from build123d import *

# Parameters (mm, degrees)
F0_W     = 380
F0_H     = 380
F1_DEPTH = 380
F2_W     = 342
F2_H     = 342
F3_DEPTH = 361
F4_W     = 40
F4_H     = 40
F5_DEPTH = 150


with BuildPart() as f1:
    # F0 (on Top) → F1 (new body)
    with BuildSketch(Plane.XY):
        Rectangle(F0_W, F0_H)
    extrude(amount=F1_DEPTH)

    # F2 (on face) → F3 (cut)
    with BuildSketch(Plane(origin=(-190, 0, 0), x_dir=(0, -1, 0), z_dir=(-1, 0, 0))):
        with Locations((0, 190)):
            Rectangle(F2_W, F2_H)
    extrude(amount=-F3_DEPTH, mode=Mode.SUBTRACT)

    # F4 (on face) → F5 (join)
    with BuildSketch(Plane(origin=(0, 0, 0), x_dir=(1, 0, 0), z_dir=(0, 0, -1))):
        with Locations((170, 170)):
            Rectangle(F4_W, F4_H)
        with Locations((-170, 170)):
            Rectangle(F4_W, F4_H)
        with Locations((-170, -170)):
            Rectangle(F4_W, F4_H)
        with Locations((170, -170)):
            Rectangle(F4_W, F4_H)
    extrude(amount=F5_DEPTH)


solid = f1.part
Source: CAD feature listing. Evaluate the final solid. Frame: model axes, mm. A direction names the side the tool comes from. Give positions to 0.01 mm unless a question says otherwise; leave off trailing zeros. Write each loop counter-clockwise with the first axis right and the second up, starting at its lowest first coordinate (ties: lowest second). Pieces come first, ordered by that corner, then holes. Notation, with made-up numbers: M 34,1 L 91,1 A26 ccw 91,26 Z; hole C 16,57.5 d10. An arc over 180 degrees is marked long. Answer as a JSON object with one key per item and string values.
Q1. Contact query for flat-ended pins moving along their axis: P1, Ø1, axis at y = -9.5, z = 195.5, coming from the -X side; P2, Ø3, axis at x = 116, y = -54.5, coming from the -Z side. Output: stop coordinate, or through.
Geometry check:
{"P1": "stops at x = 171", "P2": "stops at z = 0"}
Q2. Ray query, line 1 along Y through (x, z) = (152.5, 319); line 2 along X through (y, z) = (-154, -49.5); line 3 along Z through (x, y) = (-108, 165.5). Return the intervals inside material, ascending.
Geometry check:
{"line 1": "y = -190 to -171, 171 to 190", "line 2": "x = -190 to -150, 150 to 190", "line 3": "z = 0 to 19, 361 to 380"}
Q3. Cut plane D-D, the plane z = 295. Return the cut outline in (x, y), then the cut area to 3 significant figures.
Geometry check:
{"outline": "M -190,-190 L 190,-190 L 190,190 L -190,190 L -190,171 L 171,171 L 171,-171 L -190,-171 Z", "area": "20,900 mm^2"}
Q4. Cut plane A-A, the plane z = -84.5. Return the cut outline in (x, y).
Geometry check:
{"outline": "M -190,-190 L -150,-190 L -150,-150 L -190,-150 Z; M -190,150 L -150,150 L -150,190 L -190,190 Z; M 150,-190 L 190,-190 L 190,-150 L 150,-150 Z; M 150,150 L 190,150 L 190,190 L 150,190 Z"}
Q5. Cut plane B-B, the plane x = 99.5. Return the cut outline in (y, z), then the cut area to 3 significant figures.
Geometry check:
{"outline": "M -190,0 L 190,0 L 190,380 L -190,380 Z; hole M -171,19 L 171,19 L 171,361 L -171,361 Z", "area": "27,400 mm^2"}
Q6. Access query for faces 4 (the face through (-12, 2, 361)), 5 (the face through (-150, 170, -74)), 6 (the face through (170, 150, -74)), 7 (the face through (190, 3, 178)). Directions: +Z, -Z, +X, -X, +Y, -Y. A direction counts if a zero-diameter tool reaches every point of the face in a straight line with its end or side. Return the directions, or none.
Geometry check:
{"face 4": "-X", "face 5": "-Z, +Y, -Y", "face 6": "-Z, +X, -X", "face 7": "+Z, -Z, +X, +Y, -Y"}
Q7. Mould query, pull axis Y, two halves, no side actions, for faces 1 (the face through (-3, -190, 178)), 2 (the face through (170, -150, -74)), 3 (the face through (-170, 170, -150)). Classes: +Y half, -Y half, draft (parallel to the pull), parting line (faces both ways), or undercut.
Geometry check:
{"face 1": "-Y half", "face 2": "undercut", "face 3": "draft"}
Q8. Cut plane C-C, the plane y = 157.5. Return the cut outline in (x, z).
Geometry check:
{"outline": "M -190,-150 L -150,-150 L -150,0 L 150,0 L 150,-150 L 190,-150 L 190,380 L -190,380 L -190,361 L 171,361 L 171,19 L -190,19 Z"}
